Design review of the part built by this model. Coordinates are the model's own, in mm. A direction names the side the tool comes from. Coordinates: 2 decimals unless noted, no trailing zeros. Loops run counter-clockwise (first coordinate to the right, second up) from the corner with the lowest first, then second, coordinate; pieces in that order, holes last. Notation, with made-up numbers: (-16, -20) - (-2, -20) arc R28 ccw to (-2, 15) - close; hole circle Ø3 at (74.5, 25.5). An arc over 180 degrees is marked (long way). Answer in a Markdown table with one row per item. Add a question column.
(1) The part is to be moulded in two halves that separate along Z. For faces 1 (the face through (-29, 3, -12.577)), 2 (the face through (34, 3, 9.648)), 3 (the face through (28, 3, -3.052)), 4 (the face through (41.952, 3, 7)), say which applies: released by +Z, released by -Z, zero draft, split by the parting line, or undercut.
(2) We need section B-B, the plane z = -6.5. Write out the cut boundary in (x, y), plus the area to 3 significant figures.
(3) To check wall thickness, follow L1, parallel to Z at x = 36, y = 6; L2, parallel to Z at x = -28, y = 2.75; L3, parallel to X at y = 5.25, z = 8.5. State the ranges of each line that lie inside material, in increasing order. Write a range as [from, to].
(4) We need section A-A, the plane x = 31.5. Write out the cut boundary in (y, z), plus the area to 3 significant figures.
(5) We need section C-C, the plane y = 3.25. Write out the cut boundary in (x, z), plus the area to 3 significant figures.
(6) We need section D-D, the plane x = -23. Write out the cut boundary in (y, z).
(7) Clearance check with flat-ended pins moving along their axes: pin 1 (1.9 mm diameter, centred on x = -25, y = 3.5, fed in from -Z); pin 2 (1.9 mm diameter, centred on x = 34.5, y = 4, fed in from -Z); pin 3 (3 mm diameter, centred on x = 35, y = 1.5, fed in from +Z). State where each tip first meets the part, or that it passes through.
(8) For faces 5 (the face through (-29, 3, 12.823)), 6 (the face through (34, 3, -9.402)), 7 (the face through (28, 3, 3.298)), list the 3-axis set-ups (+Z, -Z, +X, -X, +Y, -Y) from which the entire face can be reached by the end or side of a thin tool; tool diameter is ignored.
from build123d import *

# Parameters (mm, degrees)
BOSS_EXTRUDE1_DEPTH = 6.35


with BuildPart() as part:
    # Sketch1 → Boss-Extrude1 (new body)
    with BuildSketch(Plane(origin=(0, 0, 0), x_dir=(1, 0, 0), z_dir=(0, 1, 0))):
        with BuildLine():
            Line((-33.137943546, 12.576818285), (-39.487943546, 12.576818285))
            Line((-39.487943546, 12.576818285), (-39.487943546, -12.823181715))
            Line((-39.487943546, -12.823181715), (-33.137943546, -12.823181715))
            Line((-33.137943546, -12.823181715), (-17.921975594, -12.823181715))
            ThreePointArc((-17.921975594, -12.823181715), (5.176532213, -24.877142303), (26.316962394, -9.648181715))
            Line((26.316962394, -9.648181715), (41.951577839, -9.648181715))
            Line((41.951577839, -9.648181715), (41.951577839, -3.298181715))
            Line((41.951577839, -3.298181715), (14.07573237, -3.298181715))
            ThreePointArc((14.07573237, -3.298181715), (-7.737943546, -0.123181715), (14.07573237, 3.051818285))
            Line((14.07573237, 3.051818285), (41.951577839, 3.051818285))
            Line((41.951577839, 3.051818285), (41.951577839, 9.401818285))
            Line((41.951577839, 9.401818285), (26.316962394, 9.401818285))
            ThreePointArc((26.316962394, 9.401818285), (5.176532213, 24.630778874), (-17.921975594, 12.576818285))
            Line((-17.921975594, 12.576818285), (-33.137943546, 12.576818285))
        make_face()
    extrude(amount=BOSS_EXTRUDE1_DEPTH)


solid = part.part
Responses:
| question | item | result |
|---|---|---|
| 1 | face 1 | released by -Z |
| 1 | face 2 | released by +Z |
| 1 | face 3 | undercut |
| 1 | face 4 | zero draft |
| 2 | outline | (-39.49, 0) - (-5.55, 0) - (-5.55, 6.35) - (-39.49, 6.35) - close; (12.35, 0) - (41.95, 0) - (41.95, 6.35) - (12.35, 6.35) - close |
| 2 | area | 403 mm2 |
| 3 | L1 | z = [-9.4, -3.05], [3.3, 9.65] |
| 3 | L2 | z = [-12.58, 12.82] |
| 3 | L3 | x = [-39.49, -3.94], [10.74, 41.95] |
| 4 | outline | (0, -9.4) - (6.35, -9.4) - (6.35, -3.05) - (0, -3.05) - close; (0, 3.3) - (6.35, 3.3) - (6.35, 9.65) - (0, 9.65) - close |
| 4 | area | 80.6 mm2 |
| 5 | outline | (-39.49, -12.58) - (-17.92, -12.58) arc R24.82 ccw to (26.32, -9.4) - (41.95, -9.4) - (41.95, -3.05) - (14.08, -3.05) arc R11.14 cw (long way) to (14.08, 3.3) - (41.95, 3.3) - (41.95, 9.65) - (26.32, 9.65) arc R24.82 ccw to (-17.92, 12.82) - (-39.49, 12.82) - close |
| 5 | area | 2,130 mm2 |
| 6 | outline | (0, -12.58) - (6.35, -12.58) - (6.35, 12.82) - (0, 12.82) - close |
| 7 | pin 1 | stops at z = -12.58 |
| 7 | pin 2 | stops at z = -9.4 |
| 7 | pin 3 | stops at z = 9.65 |
| 8 | face 5 | +Z, -X, +Y, -Y |
| 8 | face 6 | -Z, +X, +Y, -Y |
| 8 | face 7 | +X, +Y, -Y |
